Build history of the part. All positions in model axes, mm. A direction names the side the tool comes from. Coordinates: 2 decimals unless noted, no trailing zeros. Write each loop counter-clockwise with the first axis right and the second up, starting at its lowest first coordinate (ties: lowest second). Pieces come first, ordered by that corner, then holes.
from build123d import *

# Parameters (mm, degrees)
SALIENTE_EXTRUIR1_DEPTH = 2
CROQUIS3_W              = 3
CROQUIS3_H              = 4
CROQUIS3_R              = 0.75
SALIENTE_EXTRUIR2_DEPTH = 2


with BuildPart() as part:
    # Croquis1 → Saliente-Extruir1 (new body)
    with BuildSketch(Plane.XY):
        with BuildLine():
            Line((0, 0), (0, -18))
            add(Edge.make_bspline(
                [(0, -18), (0.591537416, -19.861671452), (3, -19)],
                knots=[0, 0, 0, 1, 1, 1], degree=2))
            ThreePointArc((3, -19), (3.639206917, -19.302348338), (3.336858579, -19.941555255))
            add(Edge.make_bspline(
                [(-1, -18.155053134), (-0.975859651, -18.232741401), (-0.899448228, -18.466363972), (-0.756134802, -18.817826734), (-0.454907757, -19.317869663), (0.02797097, -19.792887209), (0.777302206, -20.197268894), (2.276173322, -20.352435091), (3.336858579, -19.941555255)],
                knots=[-0.039688193, -0.039688193, -0.039688193, 0.009047191, 0.057782575, 0.155253343, 0.285214367, 0.415175391, 0.610116928, 1, 1, 1], degree=2))
            Line((-1, -18.155053134), (-1, 0))
            ThreePointArc((-1, 0), (-0.5, 0.5), (0, 0))
        make_face()
    extrude(amount=SALIENTE_EXTRUIR1_DEPTH)

    # Croquis3 → Saliente-Extruir2 (add)
    with BuildSketch(Plane(origin=(0, 0, 0), x_dir=(-1, 0, 0), z_dir=(0, 0, -1))):
        with Locations((-1.5, -6)):
            Rectangle(CROQUIS3_W, CROQUIS3_H)
        with Locations((-1.5, -6)):
            Circle(CROQUIS3_R, mode=Mode.SUBTRACT)
    extrude(amount=-SALIENTE_EXTRUIR2_DEPTH)


solid = part.part
(1) 3-axis set-ups, long thin cutter, end or side, ignore diameter. For faces 1 (the flat face through (-0.2, -9.8, 2)), 2 (the flat face through (0, -2, 1)), 3 (the flat face through (0, -13, 1)): which of +Z, -Z, +X, -X, +Y, -Y reach the whole face in a straight line?
(2) Two-plate mould, pull along Y, no slides. Class faces 4 (the flat face through (-0.2, -9.8, 0)), 5 (the flat face through (2, -8, 1)), 6 (the cylindrical face through (-0.5, 0.5, 1)): pulls with the +Y half, pulls with the -Y half, needs draft (parallel to the pull), parting line crosses it, or undercut.
(3) Probe L1, parallel to Y at x = 1.5, z = 1.4; L2, parallel to X at y = -9.25, z = 1.9; L3, parallel to Y at x = 2.15, z = 1.4. List the from-to ranges inside material, lowest first.
(4) Slice it at A-A, the plane y = -6. List the corners of the cut face in (x, z), and give its area (3 significant figures).
(5) Slice it at B-B, the plane y = -2.5. List the corners of the cut face in (x, z), and give its area (3 significant figures).
(6) Slice it at C-C, the plane x = 1.1. Give the number of separate pieces and of enclosed holes in the cut face, and give its area (3 significant figures).
(7) Flat gauge pins, fed straight in: P1, Ø1.5, axis at x = 2, y = -15.5, coming from the -Z side; P2, Ø0.6, axis at y = -5.5, z = 0.5, coming from the +X side. Where does each tip first touch, or does it go through?
Results:
1. face 1: +Z, +X, -X, +Y, -Y
1. face 2: +Z, -Z, +X, +Y
1. face 3: +Z, -Z, +X
2. face 4: needs draft
2. face 5: undercut
2. face 6: pulls with the +Y half
3. L1: y = -20.27 to -19.27, -8 to -6.75, -5.25 to -4
3. L2: x = -1 to 0
3. L3: y = -20.24 to -19.23, -8 to -6.37, -5.63 to -4
4. outline: (-1, 0) - (0.75, 0) - (0.75, 2) - (-1, 2) - close; (2.25, 0) - (3, 0) - (3, 2) - (2.25, 2) - close
4. area: 5.00 mm2
5. outline: (-1, 0) - (0, 0) - (0, 2) - (-1, 2) - close
5. area: 2.00 mm2
6. separate pieces: 3
6. enclosed holes: 0
6. area: 7.52 mm2
7. P1: passes through
7. P2: stops at x = 3
